Autodesk Inventor part; units mm, degrees
ref_plane "YZ Plane" through (0, 0, 0) normal (1, 0, 0) x (0, 1, 0)
ref_plane "XZ Plane" through (0, 0, 0) normal (0, 1, 0) x (-1, 0, 0)
ref_plane "XY Plane" through (0, 0, 0) normal (0, 0, 1) x (1, 0, 0)
sketch "Sketch1" plane through (0, 0, 0) normal (0, 1, 0) x (-1, 0, 0)
  circle A0 centre (0, -34) radius 6
  circle A1 centre (0, 34) radius 6
  arc A2 (14.5606, -27.3676) -> (14.3587, -41.0588) centre (0, -34) ccw construction
  circle A3 centre (0, 34) radius 16 construction
  circle A4 centre (0, 0) radius 31 construction
  arc A5 (27.82, -13.6765) -> (27.82, 13.6765) centre (0, 0) ccw
  arc A6 (14.3587, 41.0588) -> (0, 50) centre (0, 34) ccw
  line L0 (27.82, 13.6765) -> (14.3587, 41.0588)
  arc A7 (0, -50) -> (14.3587, -41.0588) centre (0, -34) ccw
  line L1 (14.3587, -41.0588) -> (27.82, -13.6765)
  line L2 (0, 34) -> (0, -34) construction
  arc A8 (-27.82, 13.6765) -> (-27.82, -13.6765) centre (0, 0) ccw
  arc A9 (0, 50) -> (-14.3587, 41.0588) centre (0, 34) ccw
  line L3 (-27.82, 13.6765) -> (-14.3587, 41.0588)
  arc A10 (-14.3587, -41.0588) -> (0, -50) centre (0, -34) ccw
  line L4 (-14.3587, -41.0588) -> (-27.82, -13.6765)
  circle A11 centre (0, 0) radius 10
  point P0 (-14.5606, -27.3676)
  dimension "d0" = 12
  dimension "d1" = 68
  dimension "d2" = 34
  dimension "d3" = 32
  dimension "d4" = 62
  dimension "d5" = 20
extrude "Extrusion1" add sketch "Sketch1" along normal mid plane 15
properties part number "base_obj5"
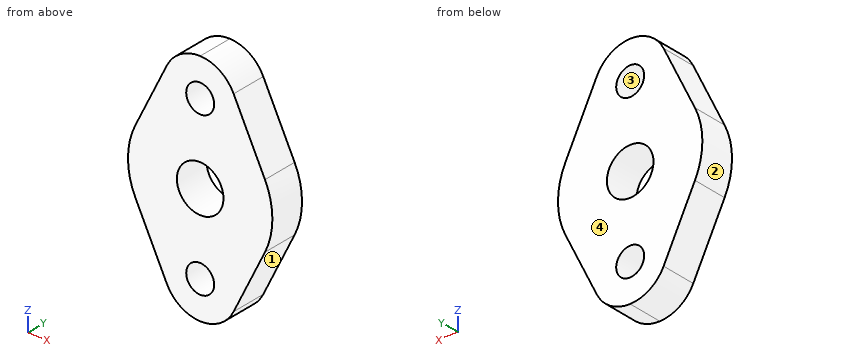
Read the model definition and answer for the solid it produces. Units are mm, in the model's axes. Face numbers are marked on the shaded views. Give positions to 0.01 mm unless a question says otherwise; leave off trailing zeros. Write each loop counter-clockwise with the first axis right and the second up, starting at its lowest first coordinate (ties: lowest second). Pieces come first, ordered by that corner, then holes. Notation, with made-up numbers: (7, 34) - (62, 34) arc R16 cw to (62, 48) - close; hole circle Ø4 at (52.25, 44). An arc over 180 degrees is marked (long way). Write item = value, one per line. Start each with the question number.
Item 1: Each of these flat-tipped pins is pushed along its axis until it touches: P1, Ø4, axis at y = -5, z = -21, coming from the +X side; P2, Ø6, axis at y = -3, z = 13.5, coming from the +X side; P3, Ø11, axis at x = 0, z = -34, coming from the +Y side; P4, Ø5, axis at x = -15.5, y = 1, coming from the -Z side. Where does it stop, or does it pass through?
Item 2: Find the intervals of material crossed by probe 1 along Z at (x, y) = (0, -1.25); probe 2 along Z at (x, y) = (-2.5, 4); probe 3 along X at (y, z) = (-5.25, 7.5), in increasing order. Write a range as [from, to].
Item 3: Find section B-B (y = -3.75). Give the vertices of the cut face in (x, z).
Item 4: Find section D-D (x = 21.5). Give the vertices of the cut face in (y, z).
Item 5: Find section C-C (x = -7.5). Give the vertices of the cut face in (y, z), then the cut area to 3 significant figures.
Item 6: The mould has two halves that part along Z. Classify the marked faces 1, 2, 3 and 4: +Z half, -Z half, draft (parallel to the pull), parting line (faces both ways), or undercut.
Item 7: Find section A-A (z = 0). Give the vertices of the cut face in (x, y).
Response:
q1.P1 = 25.2
q1.P2 = 29.17
q1.P3 = through
q1.P4 = -43.33
q2.probe_1 = [-50, -40], [-28, -10], [10, 28], [40, 50]
q2.probe_2 = [-49.8, -39.45], [-28.55, -9.68], [9.68, 28.55], [39.45, 49.8]
q2.probe_3 = [-30.08, -6.61], [6.61, 30.08]
q3.outline = (-27.82, -13.68) - (-14.36, -41.06) arc R16 ccw to (0, -50) arc R16 ccw to (14.36, -41.06) - (27.82, -13.68) arc R31 ccw to (27.82, 13.68) - (14.36, 41.06) arc R16 ccw to (0, 50) arc R16 ccw to (-14.36, 41.06) - (-27.82, 13.68) arc R31 ccw to start; hole circle Ø20 at (0, 0); hole circle Ø12 at (0, -34); hole circle Ø12 at (0, 34)
q4.outline = (-7.5, -26.53) - (7.5, -26.53) - (7.5, 26.53) - (-7.5, 26.53) - close
q5.outline = (-7.5, -48.13) - (7.5, -48.13) - (7.5, -6.61) - (-7.5, -6.61) - close; (-7.5, 6.61) - (7.5, 6.61) - (7.5, 48.13) - (-7.5, 48.13) - close
q5.area = 1,250 mm²
q6.face_1 = -Z half
q6.face_2 = parting line
q6.face_3 = undercut
q6.face_4 = draft
q7.outline = (-31, -7.5) - (-10, -7.5) - (-10, 7.5) - (-31, 7.5) - close; (10, -7.5) - (31, -7.5) - (31, 7.5) - (10, 7.5) - close
